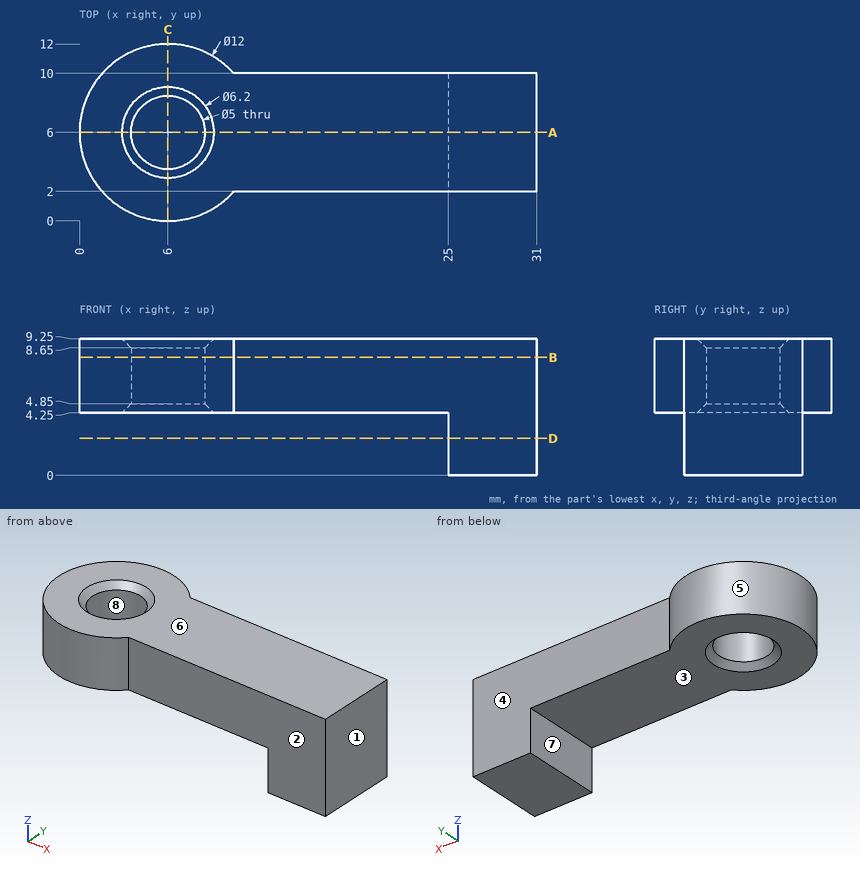
Study the drawing (mm; zero at the part's minimum x, y, z) and answer. A direction names the side the tool comes from. Coordinates: 2 decimals unless noted, no trailing zeros. Order: outer loops, then holes, each group sorted by start corner. A loop starts at its lowest first (then second) coordinate and runs counter-clockwise, first axis right, second up. Notation, with made-up numbers: (25.25, 52.25) -> (65.25, 52.25) arc R17 ccw to (65.25, 64.25) -> close; hole circle Ø5 at (-38, -38.5). An arc over 180 degrees is marked (long way). Answer in a Markdown table with one row per item. Add a question column.
Item 1: Find section B-B (z = 8). Write down the section's boundary in (x, y), then the cut area to 3 significant figures.
Item 2: Find section A-A (y = 6). Write down the section's boundary in (x, z), then the cut area to 3 significant figures.
Item 3: Find section C-C (x = 6). Write down the section's boundary in (y, z), then the cut area to 3 significant figures.
Item 4: Each of these flat-tipped pins is pushed along its axis until it touches: P1, Ø3.5, axis at y = 5.5, z = 1.5, coming from the -X side; P2, Ø4.5, axis at x = 17, z = 2.5, coming from the -Y side; P3, Ø5, axis at x = 18, y = 2, coming from the -Z side. Where does it stop, or does it pass through?
Item 5: Find the intervals of material crossed by L1, parallel to Y at x = 6, z = 6.85; L2, parallel to X at y = 6, z = 6.8; L3, parallel to Z at x = 14.5, y = 6, in increasing order. Write a range as from..to.
Item 6: Which of the six approach directions +Z, -Z, +X, -X, +Y, -Y give full straight-line access (tool end or side, diameter ignored) to the marked faces 1, 2, 3 and 4?
Item 7: Determine the mould class of the marked faces 5, 6, 7 and 8 for opening direction X: +X half, -X half, draft (parallel to the pull), parting line (faces both ways), or undercut.
Item 8: Find section D-D (z = 2.5). Write down the section's boundary in (x, y).
Result set:
| question | item | result |
|---|---|---|
| 1 | outline | (10.47, 2) -> (31, 2) -> (31, 10) -> (10.47, 10) arc R6 ccw (long way) to start; hole circle Ø5 at (6, 6) |
| 1 | area | 249 mm² |
| 2 | outline | (0, 4.25) -> (2.9, 4.25) -> (3.5, 4.85) -> (3.5, 8.65) -> (2.9, 9.25) -> (0, 9.25) -> close; (8.5, 4.85) -> (9.1, 4.25) -> (25, 4.25) -> (25, 0) -> (31, 0) -> (31, 9.25) -> (9.1, 9.25) -> (8.5, 8.65) -> close |
| 2 | area | 155 mm² |
| 3 | outline | (0, 4.25) -> (2.9, 4.25) -> (3.5, 4.85) -> (3.5, 8.65) -> (2.9, 9.25) -> (0, 9.25) -> close; (8.5, 4.85) -> (9.1, 4.25) -> (12, 4.25) -> (12, 9.25) -> (9.1, 9.25) -> (8.5, 8.65) -> close |
| 3 | area | 34.3 mm² |
| 4 | P1 | stops at x = 25 |
| 4 | P2 | stops at y = 2 |
| 4 | P3 | stops at z = 4.25 |
| 5 | L1 | y = 0..3.5, 8.5..12 |
| 5 | L2 | x = 0..3.5, 8.5..31 |
| 5 | L3 | z = 4.25..9.25 |
| 6 | face 1 | +Z, -Z, +X, +Y, -Y |
| 6 | face 2 | +Z, -Z, +X, -Y |
| 6 | face 3 | -Z, -X, +Y, -Y |
| 6 | face 4 | +Z, -Z, +X, +Y |
| 7 | face 5 | parting line |
| 7 | face 6 | draft |
| 7 | face 7 | -X half |
| 7 | face 8 | undercut |
| 8 | outline | (25, 2) -> (31, 2) -> (31, 10) -> (25, 10) -> close |
